Input: dimensioned drawing with shaded views. Units: mm. Origin: part minimum x, y, z. Coordinates: 2 decimals unless noted, no trailing zeros. Loops run counter-clockwise (first coordinate to the right, second up) from the corner with the lowest first, then second, coordinate; pieces in that order, holes last.
Item 1: Section B-B on z = 160.5. Return loops of the section in (x, y).
Item 2: Section A-A on x = 308.61. Return loops of the section in (y, z) (1 decimal), and give its area (3 significant figures).
Item 3: Section C-C on y = 7.75. Give the number of separate pieces and of enclosed holes in the cut face, and give its area (3 significant figures).
Item 4: Ray query, line 1 along X through (y, z) = (9, 173.99) (1 decimal); line 2 along Z through (x, y) = (308.61, 8) (1 decimal); line 3 along X through (y, z) = (1.75, 67). Return the intervals inside material, ascending.
Item 5: Section D-D on x = 163.83. Return loops of the section in (y, z) (1 decimal), and give its area (3 significant figures).
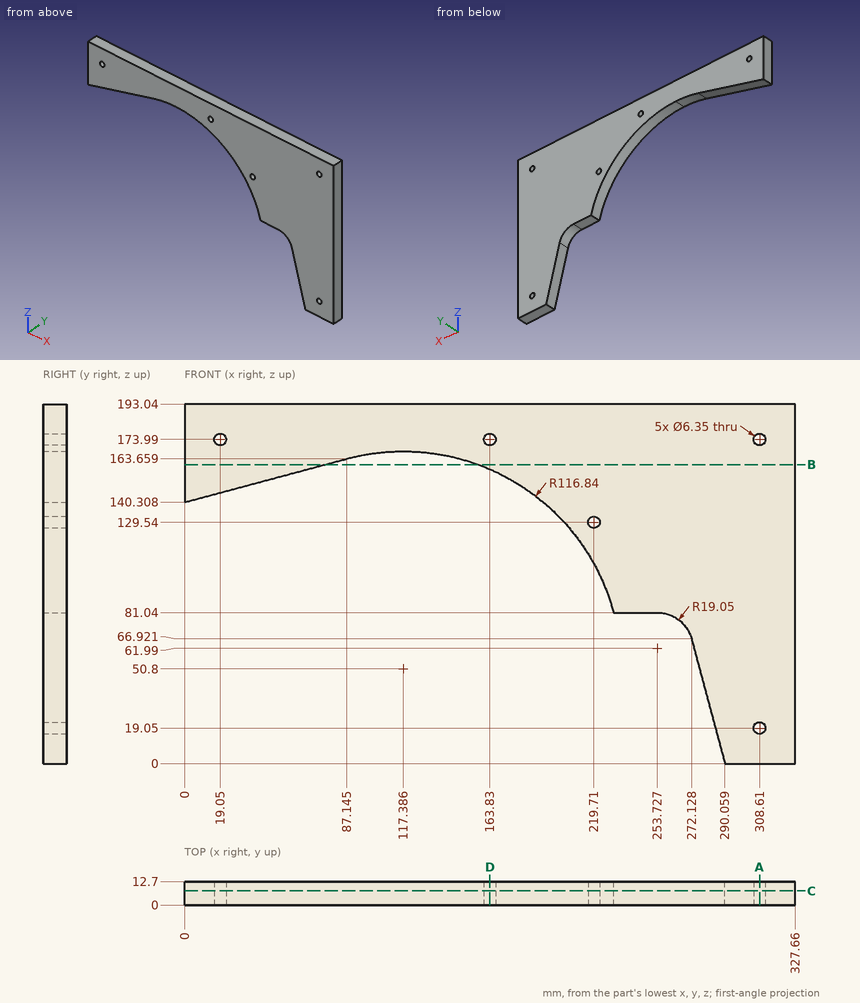
Results found:
1. outline: (0, 0) - (75.36, 0) - (75.36, 12.7) - (0, 12.7) - close; (157.6, 0) - (327.66, 0) - (327.66, 12.7) - (157.6, 12.7) - close
2. outline: (0, 0) - (12.7, 0) - (12.7, 15.9) - (0, 15.9) - close; (0, 22.2) - (12.7, 22.2) - (12.7, 170.8) - (0, 170.8) - close; (0, 177.2) - (12.7, 177.2) - (12.7, 193) - (0, 193) - close
2. area: 2,290 mm2
3. separate pieces: 1
3. enclosed holes: 5
3. area: 24,500 mm2
4. line 1: x = 0 to 15.9, 22.2 to 160.7, 167 to 305.4, 311.8 to 327.7
4. line 2: z = 0 to 15.9, 22.2 to 170.8, 177.2 to 193
4. line 3: x = 272.11 to 327.66
5. outline: (0, 158) - (12.7, 158) - (12.7, 170.8) - (0, 170.8) - close; (0, 177.2) - (12.7, 177.2) - (12.7, 193) - (0, 193) - close
5. area: 364 mm2
